Drawing for the job (mm, zero at the part's lowest x, y, z). Give positions to 0.01 mm unless a question says otherwise; leave off trailing zeros. Order: outer loops, then holes, each group sorted by start corner. A loop starts at its lowest first (then second) coordinate and runs counter-clockwise, first axis right, second up. Notation, with made-up numbers: (79, -11.5) - (124, -11.5) arc R34 cw to (124, 19.5) - close; hole circle Ø5 at (54, 59). An arc over 180 degrees is marked (long way). One line per item, written item: value.
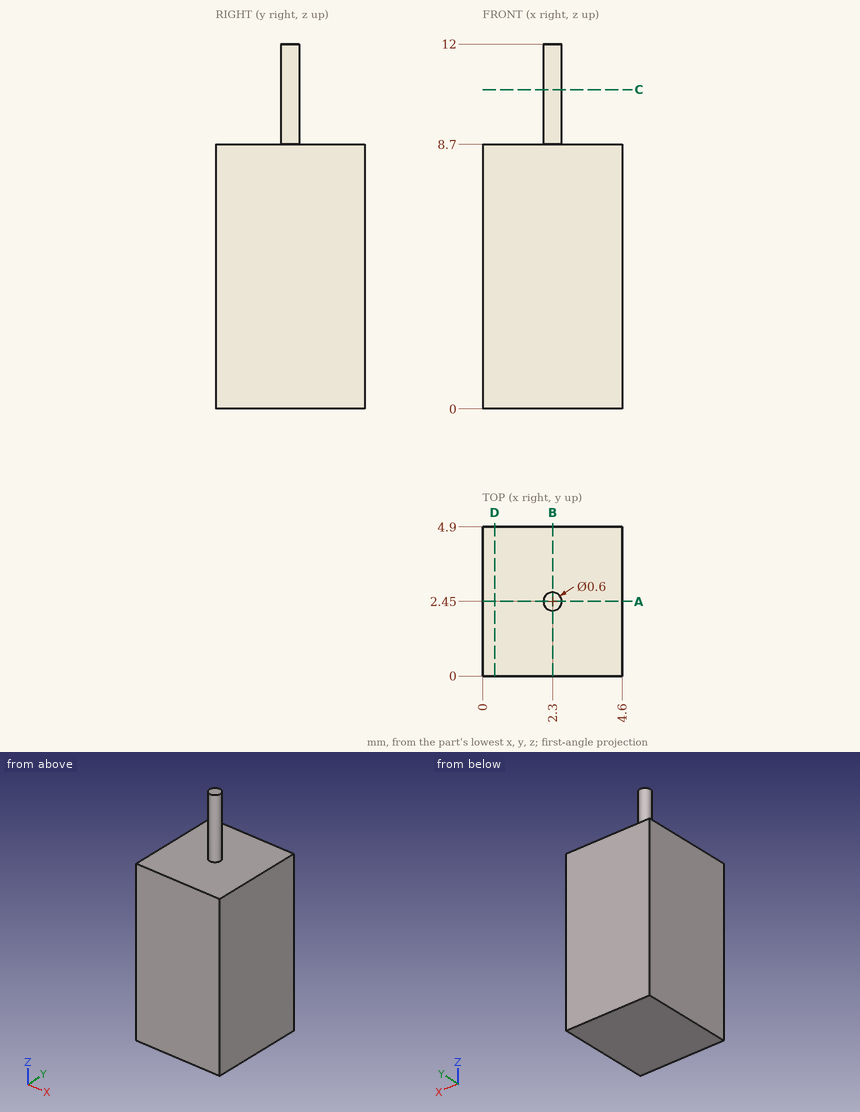
1) Pin check, flat tips, straight feed: pin 1 (1.5 mm diameter, centred on x = 2, z = 10.5, fed in from -Y); pin 2 (1.5 mm diameter, centred on x = 3, y = 4.5, fed in from +Z). Stop position of each tip, or through.
Outcome:
pin 1: stops at y = 2.15
pin 2: stops at z = 8.7
2) Drill centre lines: line 1 along Z through (x, y) = (1.75, 2.3); line 2 along Y through (x, z) = (2.1, 11.5). Where is each one in solid material? Low to high. Write a range as from..to.
Outcome:
line 1: z = 0..8.7
line 2: y = 2.23..2.67
3) Cut at C-C, the plane z = 10.5. Give the cut face in (x, y), then the cut area to 3 significant figures.
Outcome:
outline: circle Ø0.6 at (2.3, 2.45)
area: 0.283 mm^2
4) Cut at D-D, the plane x = 0.4. Give the cut face in (y, z), then the cut area to 3 significant figures.
Outcome:
outline: (0, 0) - (4.9, 0) - (4.9, 8.7) - (0, 8.7) - close
area: 42.6 mm^2
5) Cut at A-A, the plane y = 2.45. Give the cut face in (x, z), then the cut area to 3 significant figures.
Outcome:
outline: (0, 0) - (4.6, 0) - (4.6, 8.7) - (2.6, 8.7) - (2.6, 12) - (2, 12) - (2, 8.7) - (0, 8.7) - close
area: 42.0 mm^2
6) Cut at B-B, the plane x = 2.3. Give the cut face in (y, z).
Outcome:
outline: (0, 0) - (4.9, 0) - (4.9, 8.7) - (2.75, 8.7) - (2.75, 12) - (2.15, 12) - (2.15, 8.7) - (0, 8.7) - close
